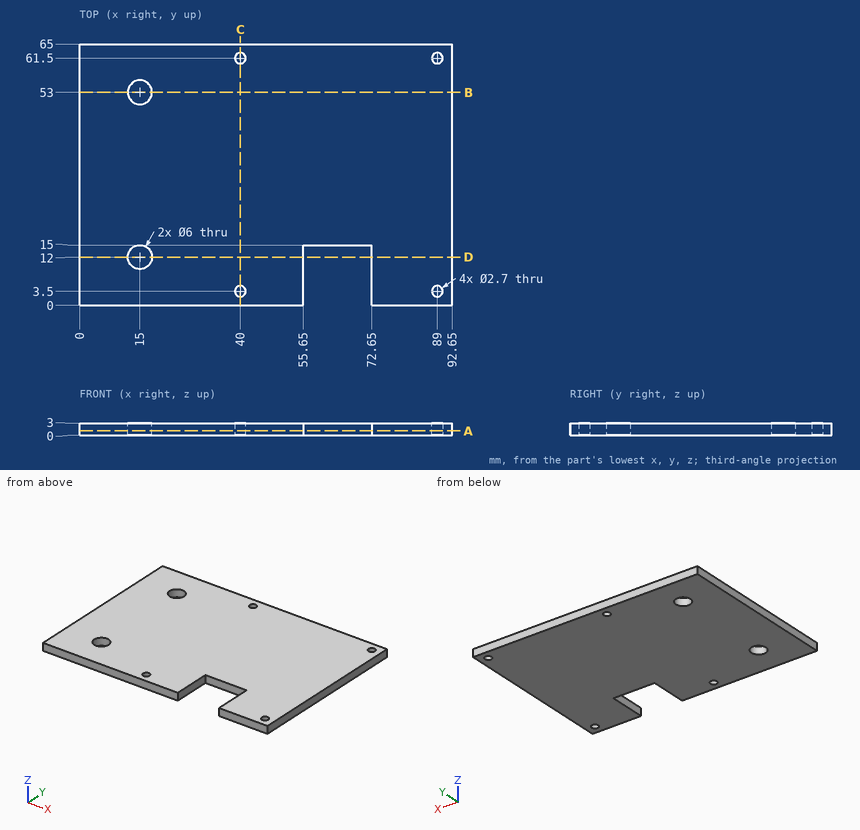
Check sheet for the drawn part. Datum: minimum x, y, z corner. Units: mm. Round coordinates to 2 decimals unless told otherwise and drop trailing zeros. Order: outer loops, then holes, each group sorted by start corner. A loop starts at its lowest first (then second) coordinate and runs counter-clockwise, first axis right, second up. Notation, with made-up numbers: (28, 69) - (67, 69) arc R11 cw to (67, 80) - close; hole circle Ø8 at (-5, 19.25). An arc over 180 degrees is marked (long way). Use a Markdown table: item, result. Add a question column.
(1) Depth check by flat-ended pin: pin 1 (3 mm diameter, centred on x = 40, y = 61.5, fed in from +Z); pin 2 (3.5 mm diameter, centred on x = 15, y = 12, fed in from -Z). Enter the tip coordinate at first touch or a pass-through.
(2) Sectioned sample at D-D, the plane y = 12. Enter the section's corners in (x, z).
(3) Sectioned sample at A-A, the plane z = 1.15. Enter the section's corners in (x, y).
(4) Material ranges on line 1 along Y through (x, z) = (15, 2.05); line 2 along Y through (x, z) = (40, 1.8); line 3 along X through (y, z) = (55.5, 1.05), recorded low to high. Write a range as [from, to].
(5) Sectioned sample at C-C, the plane x = 40. Enter the section's corners in (y, z), and give its area (3 significant figures).
(6) Sectioned sample at B-B, the plane y = 53. Enter the section's corners in (x, z), and give its area (3 significant figures).
Answers below:
| question | item | result |
|---|---|---|
| 1 | pin 1 | z = 3 |
| 1 | pin 2 | through |
| 2 | outline | (0, 0) - (12, 0) - (12, 3) - (0, 3) - close; (18, 0) - (55.65, 0) - (55.65, 3) - (18, 3) - close; (72.65, 0) - (92.65, 0) - (92.65, 3) - (72.65, 3) - close |
| 3 | outline | (0, 0) - (55.65, 0) - (55.65, 15) - (72.65, 15) - (72.65, 0) - (92.65, 0) - (92.65, 65) - (0, 65) - close; hole circle Ø6 at (15, 12); hole circle Ø6 at (15, 53); hole circle Ø2.7 at (40, 3.5); hole circle Ø2.7 at (40, 61.5); hole circle Ø2.7 at (89, 3.5); hole circle Ø2.7 at (89, 61.5) |
| 4 | line 1 | [0, 9], [15, 50], [56, 65] |
| 4 | line 2 | [0, 2.15], [4.85, 60.15], [62.85, 65] |
| 4 | line 3 | [0, 13.34], [16.66, 92.65] |
| 5 | outline | (0, 0) - (2.15, 0) - (2.15, 3) - (0, 3) - close; (4.85, 0) - (60.15, 0) - (60.15, 3) - (4.85, 3) - close; (62.85, 0) - (65, 0) - (65, 3) - (62.85, 3) - close |
| 5 | area | 179 mm² |
| 6 | outline | (0, 0) - (12, 0) - (12, 3) - (0, 3) - close; (18, 0) - (92.65, 0) - (92.65, 3) - (18, 3) - close |
| 6 | area | 260 mm² |
